Geometry: final body of the model. Coordinates: model frame, mm. A direction names the side the tool comes from. Round coordinates to 2 decimals unless told otherwise and drop trailing zeros. Write each loop counter-clockwise with the first axis right and the second up, starting at its lowest first coordinate (ties: lowest second). Pieces come first, ordered by that corner, then holes. Notation, with made-up numbers: M 47,40 L 63,40 A14 ccw 63,62 Z; hole C -28.75,37.25 d11. An arc over 180 degrees is marked long. Use one line per item in the form item = value. Start each with the question number.
from build123d import *

# Parameters (mm, degrees)
SKETCH1_W           = 23.862
SKETCH1_H           = 25
SKETCH1_R           = 1.1
BOSS_EXTRUDE1_DEPTH = 1
FILLET1_R           = 2
SKETCH2_W           = 8.5
SKETCH2_H           = 8.5
BOSS_EXTRUDE2_DEPTH = 6


with BuildPart() as part:
    # Sketch1 → Boss-Extrude1 (new body)
    with BuildSketch(Plane(origin=(0, 0, 0), x_dir=(1, 0, 0), z_dir=(0, 1, 0))):
        Rectangle(SKETCH1_W, SKETCH1_H)
        with Locations(Location((-10.02204, 10.5, 0), (0, 0, 270))):
            Circle(SKETCH1_R, mode=Mode.SUBTRACT)
        with Locations(Location((2.469, 10.5, 0), (0, 0, 270))):
            Circle(SKETCH1_R, mode=Mode.SUBTRACT)
        with Locations(Location((2.469, -10.5, 0), (0, 0, 90))):
            Circle(SKETCH1_R, mode=Mode.SUBTRACT)
        with Locations(Location((-10.02204, -10.5, 0), (0, 0, 90))):
            Circle(SKETCH1_R, mode=Mode.SUBTRACT)
    extrude(amount=BOSS_EXTRUDE1_DEPTH)

    # Fillet1
    fillet1_edges = [part.edges().sort_by_distance(p)[0] for p in [
        (11.931, 0.5, 12.5),
        (-11.931, 0.5, 12.5),
        (-11.931, 0.5, -12.5),
        (11.931, 0.5, -12.5),
    ]]
    fillet(fillet1_edges, radius=FILLET1_R)

    # Sketch2 → Boss-Extrude2 (add)
    with BuildSketch(Plane(origin=(0, 1, 0), x_dir=(1, 0, 0), z_dir=(0, 1, 0))):
        with Locations((2.469, 0)):
            Rectangle(SKETCH2_W, SKETCH2_H)
    extrude(amount=BOSS_EXTRUDE2_DEPTH)


solid = part.part
1. Ray query, probe 1 along X at (y, z) = (0.25, -10.5); probe 2 along Y at (x, z) = (9.25, 9); probe 3 along Z at (x, y) = (-0.25, 3.75). Return the intervals inside material, ascending.
2. Set-up query: faces 1 (the face through (-1.781, 4, 0)), 2 (the face through (2, 4, 4.25)), 3 (the face through (6.719, 4, 0)). Return all of +Z, -Z, +X, -X, +Y, -Y with unobstructed straight access to the full face (end or side cutting, diameter ignored); none if empty.
3. Section query B-B (z = -10). Return loops of the section in (x, y).
4. Contact query for flat-ended pins moving along their axis: pin 1 (1.5 mm diameter, centred on y = 5.5, z = -3.5, fed in from +X); pin 2 (12 mm diameter, centred on x = -6.5, z = 4, fed in from +Y); pin 3 (3 mm diameter, centred on x = -10.02, z = -10.5, fed in from +Y); pin 4 (1.8 mm diameter, centred on y = 5, z = -2, fed in from -X). Output: stop coordinate, or through.
5. Pull-direction query (Z, two-part tool) for faces 4 (the face through (11.33, 0.51, 11.93)), 5 (the face through (-11.931, 0.5, 0.1)), 6 (the face through (2.14, 0.49, 9.45)), 7 (the face through (2.048, 0.493, -9.484)); classes: released by +Z, released by -Z, zero draft, split by the parting line, or undercut.
6. Section query A-A (x = -9.25). Return loops of the section in (y, z).
7. Section query C-C (x = 5.75). Return loops of the section in (y, z).
8. Section query D-D (z = -3.5). Return loops of the section in (x, y).
Checks:
q1.probe_1 = -11.93 to -11.12, -8.92 to 1.37, 3.57 to 11.93
q1.probe_2 = 0 to 1
q1.probe_3 = -4.25 to 4.25
q2.face_1 = +Z, -Z, -X, +Y
q2.face_2 = +Z, +X, -X, +Y
q2.face_3 = +Z, -Z, +X, +Y
q3.outline = M -11.93,0 L -11,0 L -11,1 L -11.93,1 Z; M -9.04,0 L 1.49,0 L 1.49,1 L -9.04,1 Z; M 3.45,0 L 11.93,0 L 11.93,1 L 3.45,1 Z
q4.pin_1 = 6.72
q4.pin_2 = 7
q4.pin_3 = 1
q4.pin_4 = -1.78
q5.face_4 = released by +Z
q5.face_5 = zero draft
q5.face_6 = undercut
q5.face_7 = undercut
q6.outline = M 0,-12.5 L 1,-12.5 L 1,-11.28 L 0,-11.28 Z; M 0,-9.72 L 1,-9.72 L 1,9.72 L 0,9.72 Z; M 0,11.28 L 1,11.28 L 1,12.5 L 0,12.5 Z
q7.outline = M 0,-12.5 L 1,-12.5 L 1,-4.25 L 7,-4.25 L 7,4.25 L 1,4.25 L 1,12.5 L 0,12.5 Z
q8.outline = M -11.93,0 L 11.93,0 L 11.93,1 L 6.72,1 L 6.72,7 L -1.78,7 L -1.78,1 L -11.93,1 Z
